Geometry check sheet. Reference: the model listing, model coordinates, mm. A direction names the side the tool comes from. Give positions to 0.01 mm unless a question says otherwise; leave off trailing zeros. Loops run counter-clockwise (first coordinate to the right, second up) from the corner with the lowest first, then second, coordinate; pieces in that order, holes last.
1. Tool access check on faces 4 (the flat face through (2.75, 7, 55)), 5 (the flat face through (0, 70, 41)), 6 (the flat face through (0, 191, 44)), 7 (the flat face through (0, 10, 42)), 8 (the flat face through (0, 95, 50)). Record the directions out of +Z, -Z, +X, -X, +Y, -Y that give a thin tool (end or side, any length) a straight path to the whole face; none if there is none.
2. Material ranges on L1, parallel to X at y = 142, z = 43.65; L2, parallel to Y at x = -5, z = 43; L3, parallel to X at y = 0, z = 54.25, recorded low to high.
3. Cross-section at D-D, the plane y = 100. Record the cut outline in (x, z), plus the area to 3 significant figures.
4. Go/stop test with flat-tipped pins: pin 1 Ø14 at (x, z) = (3.5, 38.5) entering from +Y; pin 2 Ø4 at (x, y) = (-13.5, 33) entering from -Z; pin 3 Ø1.5 at (x, y) = (-4.5, 54) entering from +Z. Record where each tip stops, or that it passes through.
5. Cross-section at B-B, the plane y = 192. Record the cut outline in (x, z).
6. Cross-section at C-C, the plane z = 57. Record the cut outline in (x, y).
7. Release check for a two-part mould opening along X. For faces 1 (the cylindrical face through (-5.45, 194.48, 43.26)), 2 (the flat face through (15, 72, 44)), 3 (the flat face through (0, -15, 55)) record: +X half, -X half, draft (parallel to the pull), parting line (faces both ways), or undercut.
8. Cross-section at A-A, the plane x = 0. Record the cut outline in (y, z), plus the area to 3 significant figures.
from build123d import *

# Parameters (mm, degrees)
SKETCH2_W                              = 30
SKETCH2_H                              = 30
BOSS_EXTRUDE1_DEPTH                    = 60
FILLET1_R                              = 10
SKETCH3_W                              = 40
SKETCH3_H                              = 25
CUT_EXTRUDE1_DEPTH                     = 69.738635424
SKETCH6_W                              = 30
SKETCH6_H                              = 40
BOSS_EXTRUDE2_DEPTH                    = 125
SKETCH7_W                              = 30
SKETCH7_H                              = 10
BOSS_EXTRUDE3_DEPTH                    = 10
FILLET2_START                          = -16
FILLET2_DEPTH                          = 32
FILLET2_START_2                        = -15
FILLET2_2_DEPTH                        = 30
SKETCH8_W                              = 25
SKETCH8_H                              = 70
CUT_EXTRUDE2_DEPTH                     = 156.241746963
SKETCH12_W                             = 30
SKETCH12_H                             = 7.5
BOSS_EXTRUDE4_DEPTH                    = 65
SKETCH13_W                             = 20
SKETCH13_H                             = 56
SERVO_HOLE_OUTER_DEPTH                 = 6
SKETCH20_R                             = 5
BOSS_EXTRUDE5_DEPTH                    = 44
FILLET_FOR_FOREARM_MOVEMENT_DEPTH      = 212.541958013
FILLET_FOR_FOREARM_MOVEMENT_DEPTH_BACK = 212.541958013
SKETCH19_R                             = 2.5
SKETCH19_W                             = 20
SKETCH19_H                             = 41
SERVO_HOLE_INNER_DEPTH                 = 26.5
MAKE_HALF_DEPTH                        = 225.629334512
ONE_MALE_JACK_DEPTH                    = 4
CHAMFER2_SIZE                          = 0.2
MALE_JACKS_COUNT                       = 2
MALE_JACKS_PITCH                       = 24
MALE_JACKS_COUNT_DIR2                  = 3
MALE_JACKS_PITCH_DIR2                  = 27
CHAMFER2_OF_MALE_JACKS_SIZE            = 0.2
ONE_FEMALE_JACK_DEPTH                  = 5
FEMALE_JACKS_COUNT                     = 2
FEMALE_JACKS_PITCH                     = 24
FEMALE_JACKS_COUNT_DIR2                = 3
FEMALE_JACKS_PITCH_DIR2                = 27
SKETCH26_R                             = 10
MAKE_LIGHER_DEPTH                      = 60


with BuildPart() as part:
    # Sketch2 → Boss-Extrude1 (new body)
    with BuildSketch(Plane.XY):
        Rectangle(SKETCH2_W, SKETCH2_H)
        with BuildLine():
            ThreePointArc((5.25, 0), (-2.561737691, -4.582575695), (-2.75, 4.472135955))
            Line((-2.75, 4.472135955), (-2.75, 8.5))
            Line((-2.75, 8.5), (0, 8.5))
            Line((0, 8.5), (2.75, 8.5))
            Line((2.75, 8.5), (2.75, 4.472135955))
            ThreePointArc((2.75, 4.472135955), (4.582575695, 2.561737691), (5.25, 0))
        make_face(mode=Mode.SUBTRACT)
    extrude(amount=BOSS_EXTRUDE1_DEPTH)

    # Fillet1
    fillet1_edges = [part.edges().sort_by_distance(p)[0] for p in [
        (15, -15, 30),
        (-15, -15, 30),
    ]]
    fillet(fillet1_edges, radius=FILLET1_R)

    # Sketch3 → Cut-Extrude1 (cut, through all)
    with BuildSketch(Plane.ZY.offset(15)):
        with Locations((30, -2.5)):
            Rectangle(SKETCH3_W, SKETCH3_H)
    extrude(amount=-CUT_EXTRUDE1_DEPTH, mode=Mode.SUBTRACT)

    # Sketch6 → Boss-Extrude2 (add)
    with BuildSketch(Plane(origin=(0, 15, 0), x_dir=(1, 0, 0), z_dir=(0, 1, 0))):
        with Locations((0, -30)):
            Rectangle(SKETCH6_W, SKETCH6_H)
    extrude(amount=BOSS_EXTRUDE2_DEPTH)

    # Sketch7 → Boss-Extrude3 (add)
    with BuildSketch(Plane(origin=(0, 15, 0), x_dir=(1, 0, 0), z_dir=(0, 1, 0))):
        with Locations((0, -5)):
            Rectangle(SKETCH7_W, SKETCH7_H)
        with Locations((0, -55)):
            Rectangle(SKETCH7_W, SKETCH7_H)
    extrude(amount=BOSS_EXTRUDE3_DEPTH)

    # Fillet2: read off the stored shape, not the designer's step
    # Fillet2 outline → Fillet2 (cut)
    with BuildSketch(Plane.YZ.offset(FILLET2_START)):
        with BuildLine():
            ThreePointArc((25, 5), (23.535533906, 1.464466094), (20, 0))
            Line((20, 0), (25, 0))
            Line((25, 0), (25, 5))
        make_face()
        with BuildLine():
            Line((25, 60), (20, 60))
            ThreePointArc((20, 60), (23.535533906, 58.535533906), (25, 55))
            Line((25, 55), (25, 60))
        make_face()
    extrude(amount=FILLET2_DEPTH, mode=Mode.SUBTRACT)

    # Fillet2 2 outline → Fillet2 2 (add)
    with BuildSketch(Plane.YZ.offset(FILLET2_START_2)):
        with BuildLine():
            Line((25, 10), (25, 5))
            ThreePointArc((25, 5), (26.464466094, 8.535533906), (30, 10))
            Line((30, 10), (25, 10))
        make_face()
        with BuildLine():
            ThreePointArc((30, 50), (26.464466094, 51.464466094), (25, 55))
            Line((25, 55), (25, 50))
            Line((25, 50), (30, 50))
        make_face()
    extrude(amount=FILLET2_2_DEPTH)

    # Sketch8 → Cut-Extrude2 (cut, through all)
    with BuildSketch(Plane(origin=(15, 0, 0), x_dir=(0, 0, -1), z_dir=(1, 0, 0))):
        with Locations((-30, 105)):
            Rectangle(SKETCH8_W, SKETCH8_H)
    extrude(amount=-CUT_EXTRUDE2_DEPTH, mode=Mode.SUBTRACT)

    # Sketch12 → Boss-Extrude4 (add)
    with BuildSketch(Plane(origin=(0, 140, 0), x_dir=(1, 0, 0), z_dir=(0, 1, 0))):
        with Locations((0, -13.75)):
            Rectangle(SKETCH12_W, SKETCH12_H)
        with Locations((0, -46.25)):
            Rectangle(SKETCH12_W, SKETCH12_H)
    extrude(amount=BOSS_EXTRUDE4_DEPTH)

    # Sketch13 → Servo Hole Outer (cut)
    with BuildSketch(Plane.XY.offset(50)):
        with Locations((0, 167)):
            Rectangle(SKETCH13_W, SKETCH13_H)
    extrude(amount=-SERVO_HOLE_OUTER_DEPTH, mode=Mode.SUBTRACT)

    # Sketch20 → Boss-Extrude5 (add)
    with BuildSketch(Plane.XY.offset(44)):
        with Locations(Location((0, 178, 0), (0, 0, 90))):
            Circle(SKETCH20_R)
    extrude(amount=-BOSS_EXTRUDE5_DEPTH)

    # Sketch23 → Fillet for Forearm Movement (cut, two sides: drawn at the far end of the back side and taken through both)
    with BuildSketch(Plane(origin=(0, 0, 10), x_dir=(-1, 0, 0), z_dir=(0, 0, -1)).offset(-FILLET_FOR_FOREARM_MOVEMENT_DEPTH_BACK)):
        with BuildLine():
            Line((-15, 194.093476939), (-15, 205))
            Line((-15, 205), (15, 205))
            Line((15, 205), (15, 194.093476939))
            ThreePointArc((15, 194.093476939), (0, 200), (-15, 194.093476939))
        make_face()
    extrude(amount=FILLET_FOR_FOREARM_MOVEMENT_DEPTH + FILLET_FOR_FOREARM_MOVEMENT_DEPTH_BACK, mode=Mode.SUBTRACT)

    # Sketch19 → Servo Hole Inner (cut)
    with BuildSketch(Plane.XY.offset(44)):
        with Locations((-5.12, 192)):
            Circle(SKETCH19_R)
        with Locations(Location((5.12, 192, 0), (0, 0, 270))):
            Circle(SKETCH19_R)
        with Locations((5.12, 142)):
            Circle(SKETCH19_R)
        with Locations(Location((-5.12, 142, 0), (0, 0, 270))):
            Circle(SKETCH19_R)
        with Locations((0, 167)):
            Rectangle(SKETCH19_W, SKETCH19_H)
    extrude(amount=-SERVO_HOLE_INNER_DEPTH, mode=Mode.SUBTRACT)

    # 3DSketch2 → Make Half (cut, through all)
    with BuildSketch(Plane(origin=(-16.97773478, -20.308334844, 30), x_dir=(0.14055892995616934, 0.9900723141314359, 0), z_dir=(0, 0, 1))):
        Polygon((0, 0), (4.55547701, -32.087976668), (230.577525736, 0), (226.022048726, 32.087976668), align=None)
    extrude(amount=-MAKE_HALF_DEPTH, mode=Mode.SUBTRACT)

    # Sketch24 → One Male Jack (add)
    with BuildSketch(Plane(origin=(0, 0, 30), x_dir=(-1, 0, 0), z_dir=(0, 0, -1))):
        Polygon((13, 67), (12.707106781, 67.707106781), (12, 68), (11.292893219, 67.707106781), (11, 67), (11.292893219, 66.292893219), (12, 66), (12.707106781, 66.292893219), align=None)
    one_male_jack = extrude(amount=ONE_MALE_JACK_DEPTH)

    # Chamfer2
    chamfer2_edges = [part.edges().sort_by_distance(p)[0] for p in [
        (-12.853553391, 66.646446609, 26),
        (-12.853553391, 67.353553391, 26),
        (-12.353553391, 67.853553391, 26),
        (-11.646446609, 67.853553391, 26),
        (-11.146446609, 67.353553391, 26),
        (-11.146446609, 66.646446609, 26),
        (-11.646446609, 66.146446609, 26),
        (-12.353553391, 66.146446609, 26),
    ]]
    chamfer(chamfer2_edges, length=CHAMFER2_SIZE)

    # Male Jacks: One Male Jack 2 × 3, 3 skipped
    with Locations(*[(i * MALE_JACKS_PITCH, -j * MALE_JACKS_PITCH_DIR2, 0) for i in range(MALE_JACKS_COUNT) for j in range(MALE_JACKS_COUNT_DIR2) if (i, j) not in ((0, 0), (0, 1), (1, 0), (1, 2))]):
        add(one_male_jack)

    # Chamfer2 of Male Jacks
    chamfer2_of_male_jacks_edges = [part.edges().sort_by_distance(p)[0] for p in [
        (-12.853553391, 12.646446609, 26),
        (-12.853553391, 13.353553391, 26),
        (-12.353553391, 13.853553391, 26),
        (-11.646446609, 13.853553391, 26),
        (-11.146446609, 13.353553391, 26),
        (-11.146446609, 12.646446609, 26),
        (-11.646446609, 12.146446609, 26),
        (-12.353553391, 12.146446609, 26),
        (11.146446609, 39.646446609, 26),
        (11.146446609, 40.353553391, 26),
        (11.646446609, 40.853553391, 26),
        (12.353553391, 40.853553391, 26),
        (12.853553391, 40.353553391, 26),
        (12.853553391, 39.646446609, 26),
        (12.353553391, 39.146446609, 26),
        (11.646446609, 39.146446609, 26),
    ]]
    chamfer(chamfer2_of_male_jacks_edges, length=CHAMFER2_OF_MALE_JACKS_SIZE)

    # Sketch25 → One Female Jack (cut)
    with BuildSketch(Plane(origin=(0, 0, 30), x_dir=(-1, 0, 0), z_dir=(0, 0, -1))):
        Polygon((-12, 68.025), (-12.724784451, 67.724784451), (-13.025, 67), (-12.724784451, 66.275215549), (-12, 65.975), (-11.275215549, 66.275215549), (-10.975, 67), (-11.275215549, 67.724784451), align=None)
    one_female_jack = extrude(amount=-ONE_FEMALE_JACK_DEPTH, mode=Mode.SUBTRACT)

    # Female Jacks: One Female Jack 2 × 3, 3 skipped
    with Locations(*[(-i * FEMALE_JACKS_PITCH, -j * FEMALE_JACKS_PITCH_DIR2, 0) for i in range(FEMALE_JACKS_COUNT) for j in range(FEMALE_JACKS_COUNT_DIR2) if (i, j) not in ((0, 0), (0, 1), (1, 0), (1, 2))]):
        add(one_female_jack, mode=Mode.SUBTRACT)

    # Sketch26 → Make Ligher (cut)
    with BuildSketch(Plane.XZ.offset(-10)):
        with Locations((0, 30)):
            Circle(SKETCH26_R)
    extrude(amount=-MAKE_LIGHER_DEPTH, mode=Mode.SUBTRACT)


solid = part.part
Result:
1. face 4: +Z, -Z
1. face 5: -Z, +X, -X, +Y
1. face 6: +Z
1. face 7: -Z, +X, -X, -Y
1. face 8: +Z, +X, -X, +Y
2. L1: x = -15 to -7.62, -2.62 to 2.62, 7.62 to 15
2. L2: y = 10 to 139.5, 144.5 to 146.5, 187.5 to 189.5, 194.5 to 199.42
2. L3: x = -15 to -5.25, 5.25 to 15
3. outline: (-15, 42.5) - (15, 42.5) - (15, 50) - (-15, 50) - close
3. area: 225 mm2
4. pin 1: stops at y = 200
4. pin 2: stops at z = 30
4. pin 3: stops at z = 50
5. outline: (-15, 42.5) - (-7.62, 42.5) - (-7.62, 44) - (-10, 44) - (-10, 50) - (-15, 50) - close; (-2.62, 42.5) - (2.62, 42.5) - (2.62, 44) - (-2.62, 44) - close; (7.62, 42.5) - (15, 42.5) - (15, 50) - (10, 50) - (10, 44) - (7.62, 44) - close
6. outline: (-15, -5) arc R10 ccw to (-5, -15) - (5, -15) arc R10 ccw to (15, -5) - (15, 24.58) - (-15, 24.58) - close; hole (-2.75, 4.47) arc R5.25 ccw (long way) to (2.75, 4.47) - (2.75, 8.5) - (-2.75, 8.5) - close
7. face 1: undercut
7. face 2: +X half
7. face 3: draft
8. outline: (-15, 50) - (-5.25, 50) - (-5.25, 60) - (-15, 60) - close; (8.5, 50) - (10, 50) - (10, 40) - (70, 40) - (70, 42.5) - (146.5, 42.5) - (146.5, 44) - (139, 44) - (139, 50) - (30, 50) arc R5 cw to (25, 55) arc R5 ccw to (20, 60) - (8.5, 60) - close; (187.5, 42.5) - (200, 42.5) - (200, 50) - (195, 50) - (195, 44) - (187.5, 44) - close
8. area: 1,440 mm2
